For this review, take the finished solid that the model builds, in its own axes (mm). A direction names the side the tool comes from. Give positions to 0.01 mm unless a question says otherwise; leave off trailing zeros. Loops run counter-clockwise (first coordinate to the right, second up) from the corner with the lowest first, then second, coordinate; pieces in that order, holes last.
```python
from build123d import *

# Parameters (mm, degrees)
F1_DEPTH = 749.3
F2_T     = -2.286
F4_DEPTH = 3.175


with BuildPart() as f1:
    # F0 (on Right) → F1 (new body)
    with BuildSketch(Plane.YZ):
        Polygon((-676.275, 73.025), (0, 0), (0, 479.425), (-676.275, 479.425), align=None)
    extrude(amount=F1_DEPTH)

    # F2
    f2_openings = [f1.faces().sort_by_distance(p)[0] for p in [
        (374.65, -338.1375, 479.425),
    ]]
    offset(amount=F2_T, openings=f2_openings)

    # F3 (on face) → F4 (cut)
    with BuildSketch(Plane(origin=(0, 0, 0), x_dir=(-1, 0, 0), z_dir=(0, 1, 0))):
        Polygon((-158.75, 479.425), (-590.55, 479.425), (-590.55, 352.425), (-565.15, 352.425), (-565.15, 0), (-184.15, 0), (-184.15, 352.425), (-158.75, 352.425), align=None)
    extrude(amount=-F4_DEPTH, mode=Mode.SUBTRACT)


solid = f1.part
```
Q1. Consider section D-D on z = 131. Give the boundary of the cut face in (x, y) (3 decimals).
Answers:
outline: (0, -676.275) - (749.3, -676.275) - (749.3, 0) - (565.15, 0) - (565.15, -2.286) - (747.014, -2.286) - (747.014, -673.989) - (2.286, -673.989) - (2.286, -2.286) - (184.15, -2.286) - (184.15, 0) - (0, 0) - close
Q2. For probe 1 along X at (y, z) = (-176, 412.5); probe 2 along Y at (x, z) = (605, 391) (3 decimals); probe 3 along Y at (x, z) = (273.5, 455) (3 decimals), list the stretches that pass through material, from the lowest coordinate up.
Answers:
probe 1: x = 0 to 2.29, 747.01 to 749.3
probe 2: y = -676.275 to -673.989, -2.286 to 0
probe 3: y = -676.275 to -673.989
Q3. For pin 1 Ø0.7 at (x, y) = (169.5, -1) entering from +Z (3 decimals); pin 2 Ø1.5 at (x, y) = (266, -479.5) entering from -Z; pin 3 Ø5 at (x, z) = (510, 347.5) entering from +Y, all flat-tipped, find the tip position at first contact; note any pin that passes through.
Answers:
pin 1: stops at z = 352.425
pin 2: stops at z = 51.7
pin 3: stops at y = -673.99
Q4. Consider section A-A on z = 429. Give the boundary of the cut face in (x, y) (3 decimals), plus the area to 3 significant figures.
Answers:
outline: (0, -676.275) - (749.3, -676.275) - (749.3, 0) - (590.55, 0) - (590.55, -2.286) - (747.014, -2.286) - (747.014, -673.989) - (2.286, -673.989) - (2.286, -2.286) - (158.75, -2.286) - (158.75, 0) - (0, 0) - close
area: 5,510 mm2
Q5. Consider section C-C on y = -423.5. Give the boundary of the cut face in (x, z) (3 decimals).
Answers:
outline: (0, 45.73) - (749.3, 45.73) - (749.3, 479.425) - (747.014, 479.425) - (747.014, 48.029) - (2.286, 48.029) - (2.286, 479.425) - (0, 479.425) - close
Q6. Mouldability with a two-part tool opening along Y and no side actions: class faces 1 (the flat face through (369, -673.989, 280)), 2 (the flat face through (2.286, -343, 244)), 3 (the flat face through (656, 0, 236)), 4 (the flat face through (0, -343, 243)) as +Y half, -Y half, draft (parallel to the pull), parting line (faces both ways), or undercut.
Answers:
face 1: undercut
face 2: undercut
face 3: +Y half
face 4: draft
Q7. Consider section B-B on x = 606.5. Give the boundary of the cut face in (y, z) (3 decimals).
Answers:
outline: (-676.275, 73.025) - (0, 0) - (0, 479.425) - (-2.286, 479.425) - (-2.286, 2.546) - (-673.989, 75.077) - (-673.989, 479.425) - (-676.275, 479.425) - close
Q8. Machinability: for faces 5 (the flat face through (749.3, -343, 243)), 6 (the flat face through (369.44, -342.84, 39.32)), which of the approach directions +Z, -Z, +X, -X, +Y, -Y give a long, thin tool a straight path to every point of the face, cutting with its end or side? Answer none if there is none.
Answers:
face 5: +Z, -Z, +X, +Y, -Y
face 6: +Z
